Source: CAD feature listing. Evaluate the final solid. Frame: model axes, mm. Give positions to 0.01 mm unless a question says otherwise; leave off trailing zeros. Loops run counter-clockwise (first coordinate to the right, second up) from the corner with the lowest first, then second, coordinate; pieces in that order, holes last.
from build123d import *

# Parameters (mm, degrees)
BOSS_EXTRUDE1_DEPTH     = 19
FILLET1_R               = 10
SKETCH2_R               = 13.5
CUT_EXTRUDE1_DEPTH      = 20
TAP_DRILL_FOR_M5_TAP1_D = 4.2
M5_CLEARANCE_HOLE1_D    = 5.5
TAP_DRILL_FOR_M5_TAP2_D = 4.2
FILLET2_R               = 4
BOSS_EXTRUDE2_DEPTH     = 19
M8_CLEARANCE_HOLE1_D    = 9


with BuildPart() as part:
    # Sketch1 → Boss-Extrude1 (new body)
    with BuildSketch(Plane.XY):
        with BuildLine():
            Line((-170.200000001, 540.824594888), (-129.309401077, 470))
            Line((-129.309401077, 470), (-93, 470))
            ThreePointArc((-93, 470), (-90.878679656, 470.878679656), (-90, 473))
            Line((-90, 473), (-90, 564.25527297))
            Line((-90, 564.25527297), (-116.225329238, 607))
            Line((-116.225329238, 607), (-170.200000001, 607))
            Line((-170.200000001, 607), (-170.200000001, 540.824594888))
        make_face()
    extrude(amount=BOSS_EXTRUDE1_DEPTH)

    # Fillet1
    fillet1_edges = [part.edges().sort_by_distance(p)[0] for p in [
        (-90, 564.25527297, 9.5),
        (-129.309401077, 470, 9.5),
        (-170.200000001, 540.824594888, 9.5),
    ]]
    fillet(fillet1_edges, radius=FILLET1_R)

    # Sketch2 → Cut-Extrude1 (cut)
    with BuildSketch(Plane.XY.offset(19)):
        with Locations((-142.000000001, 577)):
            Circle(SKETCH2_R)
    extrude(amount=-CUT_EXTRUDE1_DEPTH, mode=Mode.SUBTRACT)

    # Tap Drill for M5 Tap1 (through all)
    with Locations(Plane(origin=(0, 0, 0), x_dir=(-1, 0, 0), z_dir=(0, 0, -1))):
        with Locations((119.000000001, 595), (119.000000001, 577), (165.000000001, 577), (165.000000001, 595)):
            Hole(TAP_DRILL_FOR_M5_TAP1_D / 2)

    # M5 Clearance Hole1 (through all)
    with Locations(Plane.XY.offset(19)):
        with Locations((-95, 545), (-125, 545), (-125, 475), (-95, 475), (-110, 490), (-110, 530)):
            Hole(M5_CLEARANCE_HOLE1_D / 2)

    # Tap Drill for M5 Tap2 (through all)
    with Locations(Plane.XY.offset(19)):
        with Locations((-165.570000001, 553.43), (-165.570000001, 600.57), (-118.430000001, 553.43), (-118.430000001, 600.57)):
            Hole(TAP_DRILL_FOR_M5_TAP2_D / 2)

    # Fillet2
    fillet2_edges = [part.edges().sort_by_distance(p)[0] for p in [
        (-116.225329238, 607, 9.5),
        (-170.200000001, 607, 9.5),
    ]]
    fillet(fillet2_edges, radius=FILLET2_R)

    # Sketch11 → Boss-Extrude2 (add)
    with BuildSketch(Plane.XY.offset(19)):
        with BuildLine():
            ThreePointArc((-80, 561.432106106), (-80.75234172, 566.866041212), (-82.952765074, 571.89115871))
            Line((-82.952765074, 571.89115871), (-106.530973281, 610.321336823))
            ThreePointArc((-106.530973281, 610.321336823), (-111.626593598, 615.216765438), (-118.464037729, 617))
            Line((-118.464037729, 617), (-166.200000001, 617))
            ThreePointArc((-166.200000001, 617), (-176.099494937, 612.899494937), (-180.200000001, 603))
            Line((-180.200000001, 603), (-180.200000001, 543.504086813))
            ThreePointArc((-180.200000001, 543.504086813), (-179.518516526, 538.327705911), (-177.520508076, 533.504086813))
            Line((-177.520508076, 533.504086813), (-143.743157806, 475))
            ThreePointArc((-143.743157806, 475), (-140.082903769, 471.339745962), (-135.082903769, 470))
            Line((-135.082903769, 470), (-123.535898385, 470))
            ThreePointArc((-123.535898385, 470), (-128.535898385, 471.339745962), (-132.196152423, 475))
            Line((-132.196152423, 475), (-168.860254039, 538.504086813))
            ThreePointArc((-168.860254039, 538.504086813), (-169.859258264, 540.915896362), (-170.200000001, 543.504086813))
            Line((-170.200000001, 543.504086813), (-170.200000001, 603))
            ThreePointArc((-170.200000001, 603), (-169.028427125, 605.828427125), (-166.200000001, 607))
            Line((-166.200000001, 607), (-118.464037729, 607))
            ThreePointArc((-118.464037729, 607), (-116.510482263, 606.490504411), (-115.054590744, 605.091810521))
            Line((-115.054590744, 605.091810521), (-91.476382537, 566.661632408))
            ThreePointArc((-91.476382537, 566.661632408), (-90.37617086, 564.149073659), (-90, 561.432106106))
            Line((-90, 561.432106106), (-90, 473))
            ThreePointArc((-90, 473), (-90.878679656, 470.878679656), (-93, 470))
            Line((-93, 470), (-90, 470))
            ThreePointArc((-90, 470), (-82.928932188, 472.928932188), (-80, 480))
            Line((-80, 480), (-80, 561.432106106))
        make_face()
    extrude(amount=-BOSS_EXTRUDE2_DEPTH)

    # M8 Clearance Hole1 (through all)
    with Locations(Plane(origin=(-110, 490, 0), x_dir=(-1, 0, 0), z_dir=(0, 0, -1))):
        with Locations((0, 0), (0, 40)):
            Hole(M8_CLEARANCE_HOLE1_D / 2)


solid = part.part
1) Cut plane A-A (z = 2.25). State how many separate pieces and enclosed holes the cut face has, and give its area (3 significant figures).
Checks:
separate pieces: 1
enclosed holes: 15
area: 11,600 mm2
2) Cut plane C-C (x = -110). Return loops of the section in (y, z), and give its area (3 significant figures).
Checks:
outline: (470, 0) - (485.5, 0) - (485.5, 19) - (470, 19) - close; (494.5, 0) - (525.5, 0) - (525.5, 19) - (494.5, 19) - close; (534.5, 0) - (614.15, 0) - (614.15, 19) - (534.5, 19) - close
area: 2,400 mm2
3) Cut plane B-B (y = 545). Return loops of the section in (x, z).
Checks:
outline: (-180.2, 0) - (-127.75, 0) - (-127.75, 19) - (-180.2, 19) - close; (-122.25, 0) - (-97.75, 0) - (-97.75, 19) - (-122.25, 19) - close; (-92.25, 0) - (-80, 0) - (-80, 19) - (-92.25, 19) - close
4) Ray query, probe 1 along Y at (x, z) = (-125, 9.5); probe 2 along X at (y, z) = (545, 12.25); probe 3 along Y at (x, z) = (-165, 11). Return the intervals inside material, ascending.
Checks:
probe 1: y = 470 to 472.25, 477.75 to 542.25, 547.75 to 617
probe 2: x = -180.2 to -127.75, -122.25 to -97.75, -92.25 to -80
probe 3: y = 511.82 to 551.41, 555.45 to 574.9, 579.1 to 592.9, 597.1 to 598.55, 602.59 to 617
5) Cut plane D-D (y = 587). Return loops of the section in (x, z).
Checks:
outline: (-180.2, 0) - (-151.07, 0) - (-151.07, 19) - (-180.2, 19) - close; (-132.93, 0) - (-92.22, 0) - (-92.22, 19) - (-132.93, 19) - close
6) Pull-direction query (Y, two-part tool) for faces 1 (the cylindrical face through (-143.757, 590.385, 9.633)), 2 (the flat face through (-94.58, 590.84, 9.63)), 3 (the cylindrical face through (-140.15, 471.38, 9.63)); classes: released by +Y, released by -Y, zero draft, split by the parting line, or undercut.
Checks:
face 1: undercut
face 2: released by +Y
face 3: released by -Y
7) Contact query for flat-ended pins moving along their axis: P1, Ø4, axis at x = -118.43, y = 600.57, coming from the +Z side; P2, Ø4, axis at x = -139, z = 5.5, coming from the -Y side. Output: stop coordinate, or through.
Checks:
P1: passes through
P2: stops at y = 470.19
